from build123d import *

# Parameters (mm, degrees)
SKETCH1_R           = 4.2
BOSS_EXTRUDE1_DEPTH = 7
BOSS_EXTRUDE2_DEPTH = 11
BOSS_EXTRUDE2_TAPER = 25
SKETCH5_R           = 1.65
SKETCH5_R_2         = 11
CUT_EXTRUDE1_DEPTH  = 19


with BuildPart() as part:
    # Sketch1 → Boss-Extrude1 (new body)
    with BuildSketch(Plane.XY):
        with BuildLine():
            Line((-25, 80), (25, 80))
            ThreePointArc((25, 80), (32.071067812, 77.071067812), (35, 70))
            Line((35, 70), (35, -65))
            ThreePointArc((35, -65), (32.071067812, -72.071067812), (25, -75))
            Line((25, -75), (-25, -75))
            ThreePointArc((-25, -75), (-32.071067812, -72.071067812), (-35, -65))
            Line((-35, -65), (-35, 70))
            ThreePointArc((-35, 70), (-32.071067812, 77.071067812), (-25, 80))
        make_face()
        with Locations((-20, -7.5)):
            Circle(SKETCH1_R, mode=Mode.SUBTRACT)
        with Locations((20, -7.5)):
            Circle(SKETCH1_R, mode=Mode.SUBTRACT)
        with Locations((20, -52.5)):
            Circle(SKETCH1_R, mode=Mode.SUBTRACT)
        with Locations((-20, -52.5)):
            Circle(SKETCH1_R, mode=Mode.SUBTRACT)
    extrude(amount=-BOSS_EXTRUDE1_DEPTH)

    # Sketch3 → Boss-Extrude2 (add)
    with BuildSketch(Plane.XY):
        with BuildLine():
            Line((-35, 16), (35, 16))
            Line((35, 16), (35, 70))
            ThreePointArc((35, 70), (32.071067812, 77.071067812), (25, 80))
            Line((25, 80), (-25, 80))
            ThreePointArc((-25, 80), (-32.071067812, 77.071067812), (-35, 70))
            Line((-35, 70), (-35, 16))
        make_face()
    extrude(amount=BOSS_EXTRUDE2_DEPTH, taper=BOSS_EXTRUDE2_TAPER)

    # Sketch5 → Cut-Extrude1 (cut, through all)
    with BuildSketch(Plane.XY.offset(11)):
        with Locations((-14.5, 56)):
            Circle(SKETCH5_R)
        with Locations((14.5, 56)):
            Circle(SKETCH5_R)
        with Locations((0, 56)):
            Circle(SKETCH5_R_2)
    extrude(amount=-CUT_EXTRUDE1_DEPTH, mode=Mode.SUBTRACT)


solid = part.part
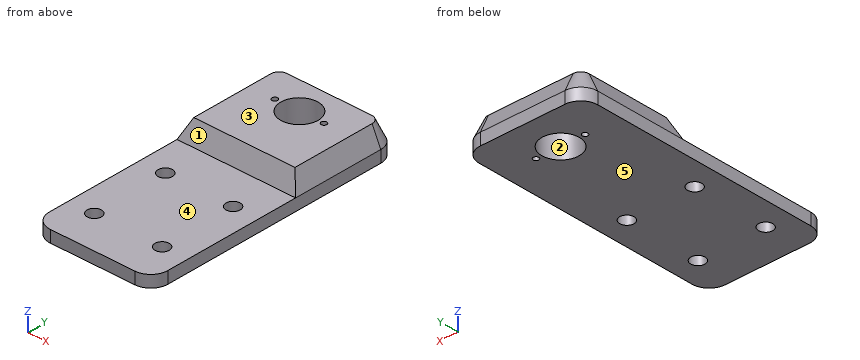
The model under review builds one solid part; all positions refer to its coordinate system, in mm. Face numbers are marked on the shaded views. A direction names the side the tool comes from. Give positions to 0.01 mm unless a question says otherwise; leave off trailing zeros. Loops run counter-clockwise (first coordinate to the right, second up) from the corner with the lowest first, then second, coordinate; pieces in that order, holes last. Notation, with made-up numbers: (60.25, 21.5) -> (113.25, 21.5) arc R28 ccw to (113.25, 54.5) -> close; hole circle Ø11 at (82.5, 31). An arc over 180 degrees is marked (long way). Write each question's results on one line, items separated by ' | '.
1) Tool access review of the marked faces 4 and 5: name each direction out of +Z, -Z, +X, -X, +Y, -Y from which nothing blocks a thin tool from reaching the whole face with its end or side.
Conclusion:
face 4: +Z, +X, -X, -Y | face 5: -Z, +X, -X, +Y, -Y
2) For line 1 along Y through (x, z) = (20, -2.25); line 2 along Y through (x, z) = (21.5, -4.75); line 3 along Y through (x, z) = (14.5, -1.5), list the stretches that pass through material, from the lowest coordinate up. Write a range as from..to.
Conclusion:
line 1: y = -75..-56.7, -48.3..-11.7, -3.3..80 | line 2: y = -75..-56.42, -48.58..-11.42, -3.58..80 | line 3: y = -75..54.35, 57.65..80
3) Insertion check: pin 1 Ø2 at (x, y) = (26, -18) entering from +Z; pin 2 Ø2 at (x, y) = (-14.5, 56) entering from -Z; pin 3 Ø8 at (x, z) = (11.5, 7) entering from +Y; pin 4 Ø3 at (x, z) = (17.5, 4) entering from -Y. Each pin has a flat end and moves straight along its axis. Give the tip position at first contact, or say it passes through.
Conclusion:
pin 1: stops at z = 0 | pin 2: passes through | pin 3: stops at y = 78.6 | pin 4: stops at y = 17.17
4) Draft analysis for pull direction Y (two halves, no side actions). For the marked faces 1, 2 and 3, state which applies: pulls with the +Y half, pulls with the -Y half, needs draft (parallel to the pull), parting line crosses it, or undercut.
Conclusion:
face 1: pulls with the -Y half | face 2: undercut | face 3: needs draft
5) Take a section at B-B, the plane y = -7.5. Give the boundary of the cut face in (x, z), plus the area to 3 significant figures.
Conclusion:
outline: (-35, -7) -> (-24.2, -7) -> (-24.2, 0) -> (-35, 0) -> close; (-15.8, -7) -> (15.8, -7) -> (15.8, 0) -> (-15.8, 0) -> close; (24.2, -7) -> (35, -7) -> (35, 0) -> (24.2, 0) -> close | area: 372 mm^2
6) Take a section at D-D, the plane x = 0. Give the boundary of the cut face in (y, z).
Conclusion:
outline: (-75, -7) -> (45, -7) -> (45, 11) -> (21.13, 11) -> (16, 0) -> (-75, 0) -> close; (67, -7) -> (80, -7) -> (80, 0) -> (74.87, 11) -> (67, 11) -> close
7) Take a section at C-C, the plane z = -1.75. Give the boundary of the cut face in (x, y).
Conclusion:
outline: (-35, -65) arc R10 ccw to (-25, -75) -> (25, -75) arc R10 ccw to (35, -65) -> (35, 70) arc R10 ccw to (25, 80) -> (-25, 80) arc R10 ccw to (-35, 70) -> close; hole circle Ø8.4 at (-20, -52.5); hole circle Ø8.4 at (-20, -7.5); hole circle Ø3.3 at (-14.5, 56); hole circle Ø22 at (0, 56); hole circle Ø3.3 at (14.5, 56); hole circle Ø8.4 at (20, -52.5); hole circle Ø8.4 at (20, -7.5)
8) Take a section at A-A, the plane x = -20. Give the boundary of the cut face in (y, z), plus the area to 3 significant figures.
Conclusion:
outline: (-75, -7) -> (-56.7, -7) -> (-56.7, 0) -> (-75, 0) -> close; (-48.3, -7) -> (-11.7, -7) -> (-11.7, 0) -> (-48.3, 0) -> close; (-3.3, -7) -> (80, -7) -> (80, 0) -> (74.87, 11) -> (21.13, 11) -> (16, 0) -> (-3.3, 0) -> close | area: 1,610 mm^2
